The model under review builds one solid part; all positions refer to its coordinate system, in mm. Face numbers are marked on the shaded views. A direction names the side the tool comes from. Give positions to 0.01 mm unless a question says otherwise; leave off trailing zeros. Write each loop counter-clockwise with the first axis right and the second up, starting at its lowest first coordinate (ties: lowest second). Pieces come first, ordered by that corner, then holes. Notation, with made-up numbers: M 53,-18.5 L 62,-18.5 A5 ccw 62,-11.5 Z; hole C -4,-33 d4. An arc over 180 degrees is marked long. Write item = value, one per line. Start each with the question number.
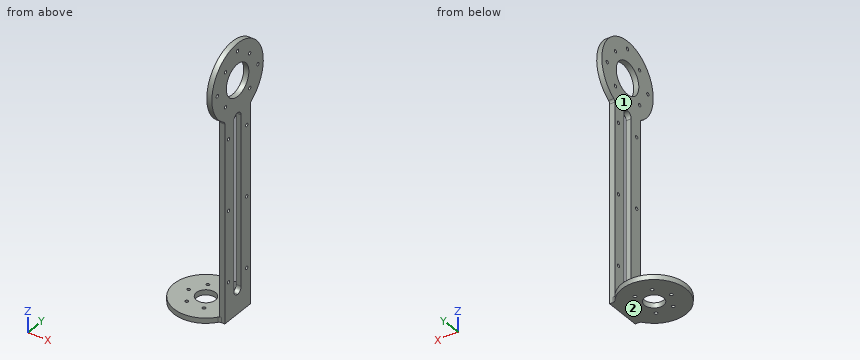
```python
from build123d import *

# Parameters (mm, degrees)
SKETCH_1_R          = 28.5
EXTRUDE_1_DEPTH     = 4
SKETCH_2_R          = 1.25
CUT_EXTRUDE_2_DEPTH = 4
CUT_EXTRUDE_START   = -4
CUT_EXTRUDE_4_DEPTH = 4
SKETCH_5_R          = 7.5
CUT_EXTRUDE_5_DEPTH = 4
SKETCH_6_W          = 4
SKETCH_6_H          = 28.262165522
EXTRUDE_2_DEPTH     = 140
SKETCH_7_R          = 12.5
EXTRUDE_3_DEPTH     = 4
SKETCH_8_R          = 1.25
CUT_EXTRUDE_6_DEPTH = 4
SKETCH_9_R          = 1.25
SKETCH_9_W          = 140
SKETCH_9_H          = 8
CUT_EXTRUDE_7_DEPTH = 4
FILLET_1_R          = 4
FILLET_2_R          = 4
FILLET_3_R          = 2.5


with BuildPart() as part:
    # 草图1 → 凸台-拉伸1 (new body)
    with BuildSketch(Plane.XY):
        Circle(SKETCH_1_R)
    extrude(amount=EXTRUDE_1_DEPTH)

    # 草图2 → 切除-拉伸2 (cut)
    with BuildSketch(Plane.XY.offset(4)):
        with Locations((-13.5, 0)):
            Circle(SKETCH_2_R)
        with Locations((-6.75, 11.691342951)):
            Circle(SKETCH_2_R)
        with Locations((6.75, 11.691342951)):
            Circle(SKETCH_2_R)
        with Locations((6.75, -11.691342951)):
            Circle(SKETCH_2_R)
        with Locations((-6.75, -11.691342951)):
            Circle(SKETCH_2_R)
    extrude(amount=-CUT_EXTRUDE_2_DEPTH, mode=Mode.SUBTRACT)

    # 草图4 → 切除-拉伸4 (cut)
    with BuildSketch(Plane.XY.offset(4).offset(CUT_EXTRUDE_START)):
        with BuildLine():
            ThreePointArc((20.75, -14.131082761), (-25.104780421, 0), (20.75, 14.131082761))
            Line((20.75, 14.131082761), (24.75, 14.131082761))
            ThreePointArc((24.75, 14.131082761), (-28.5, 0), (24.75, -14.131082761))
            Line((24.75, -14.131082761), (20.75, -14.131082761))
        make_face()
        with BuildLine():
            Line((24.75, 14.131082761), (24.75, 0))
            Line((24.75, 0), (28.5, 0))
            ThreePointArc((28.5, 0), (27.546551508, 7.310095759), (24.75, 14.131082761))
        make_face()
        with BuildLine():
            Line((28.5, 0), (24.75, 0))
            Line((24.75, 0), (24.75, -14.131082761))
            ThreePointArc((24.75, -14.131082761), (27.546551508, -7.310095759), (28.5, 0))
        make_face()
    extrude(amount=CUT_EXTRUDE_4_DEPTH, mode=Mode.SUBTRACT)

    # 草图5 → 切除-拉伸5 (cut)
    with BuildSketch(Plane.XY.offset(4)):
        Circle(SKETCH_5_R)
    extrude(amount=-CUT_EXTRUDE_5_DEPTH, mode=Mode.SUBTRACT)

    # 草图6 → 凸台-拉伸2 (add)
    with BuildSketch(Plane.XY.offset(4)):
        with Locations((22.75, 0)):
            Rectangle(SKETCH_6_W, SKETCH_6_H)
    extrude(amount=EXTRUDE_2_DEPTH)

    # 草图7 → 凸台-拉伸3 (add)
    with BuildSketch(Plane(origin=(24.75, 0, 0), x_dir=(0, 0, -1), z_dir=(1, 0, 0))):
        with BuildLine():
            Line((-144, 14.131082761), (-155.25, 14.131082761))
            ThreePointArc((-155.25, 14.131082761), (-208.5, 0), (-155.25, -14.131082761))
            Line((-155.25, -14.131082761), (-144, -14.131082761))
            Line((-144, -14.131082761), (-144, 14.131082761))
        make_face()
        with Locations((-180, 0)):
            Circle(SKETCH_7_R, mode=Mode.SUBTRACT)
    extrude(amount=-EXTRUDE_3_DEPTH)

    # 草图8 → 切除-拉伸6 (cut)
    with BuildSketch(Plane(origin=(24.75, 0, 0), x_dir=(0, 0, -1), z_dir=(1, 0, 0))):
        with Locations((-166.564971157, 13.435028843)):
            Circle(SKETCH_8_R)
        with Locations((-166.564971157, -13.435028843)):
            Circle(SKETCH_8_R)
        with Locations((-193.435028843, -13.435028843)):
            Circle(SKETCH_8_R)
        with Locations((-193.435028843, 13.435028843)):
            Circle(SKETCH_8_R)
    extrude(amount=-CUT_EXTRUDE_6_DEPTH, mode=Mode.SUBTRACT)

    # 草图9 → 切除-拉伸7 (cut)
    with BuildSketch(Plane(origin=(24.75, 0, 0), x_dir=(0, 0, -1), z_dir=(1, 0, 0))):
        with Locations((-140, 10.131082761)):
            Circle(SKETCH_9_R)
        with Locations((-180, 22.5)):
            Circle(SKETCH_9_R)
        with Locations((-202.5, 0)):
            Circle(SKETCH_9_R)
        with Locations((-180, -22.5)):
            Circle(SKETCH_9_R)
        with Locations((-85, 10.131082761)):
            Circle(SKETCH_9_R)
        with Locations((-30, 10.131082761)):
            Circle(SKETCH_9_R)
        with Locations(Location((-30, -10.131082761, 0), (0, 0, 180))):
            Circle(SKETCH_9_R)
        with Locations(Location((-85, -10.131082761, 0), (0, 0, 180))):
            Circle(SKETCH_9_R)
        with Locations(Location((-140, -10.131082761, 0), (0, 0, 180))):
            Circle(SKETCH_9_R)
        with Locations((-85, 0)):
            Rectangle(SKETCH_9_W, SKETCH_9_H)
    extrude(amount=-CUT_EXTRUDE_7_DEPTH, mode=Mode.SUBTRACT)

    # 圆角1
    fillet_1_edges = [part.edges().sort_by_distance(p)[0] for p in [
        (22.75, -4, 155),
        (22.75, 4, 155),
    ]]
    fillet(fillet_1_edges, radius=FILLET_1_R - 0.0001)  # a hair under: the kernel refuses the full size

    # 圆角2
    fillet_2_edges = [part.edges().sort_by_distance(p)[0] for p in [
        (22.75, 4, 15),
        (22.75, -4, 15),
    ]]
    fillet(fillet_2_edges, radius=FILLET_2_R - 0.0001)  # a hair under: the kernel refuses the full size

    # 圆角3
    fillet_3_edges = [part.edges().sort_by_distance(p)[0] for p in [
        (22.75, -14.131082761, 155.25),
        (22.75, 14.131082761, 155.25),
        (20.75, -14.131082761, 2),
        (20.75, 14.131082761, 2),
    ]]
    fillet(fillet_3_edges, radius=FILLET_3_R)


solid = part.part
```
Item 1: Clearance check with flat-ended pins moving along their axes: P1, Ø23.5, axis at x = -8.5, y = 4.5, coming from the +Z side; P2, Ø2, axis at x = 14.5, y = 1, coming from the -Z side; P3, Ø2, axis at x = 22, z = 98, coming from the -Y side; P4, Ø2, axis at y = -18, z = 163.5, coming from the -X side. State where each tip first meets the part, or that it passes through.
Item 2: We need section A-A, the plane z = 105. Write out the cut boundary in (x, y).
Item 3: For the marked faces 1 and 2, list the 3-axis set-ups (+Z, -Z, +X, -X, +Y, -Y) from which the entire face can be reached by the end or side of a thin tool; tool diameter is ignored.
Item 4: To check wall thickness, follow probe 1 along Y at (x, z) = (23.9, 85); probe 2 along X at (y, z) = (15, 179); probe 3 along Z at (x, y) = (-11, 1). State the ranges of each line that lie inside material, in increasing order. Write a range as [from, to].
Item 5: We need section C-C, the plane z = 162. Write out the cut boundary in (x, y), and give its area (3 significant figures).
Item 6: We need section B-B, the plane z = 190. Write out the cut boundary in (x, y).
Worked out:
q1.P1 = 4
q1.P2 = 0
q1.P3 = -14.13
q1.P4 = 20.75
q2.outline = M 20.75,-14.13 L 24.75,-14.13 L 24.75,-4 L 20.75,-4 Z; M 20.75,4 L 24.75,4 L 24.75,14.13 L 20.75,14.13 Z
q3.face_1 = +Z, -X, +Y, -Y
q3.face_2 = -Z, +X, -X, +Y, -Y
q4.probe_1 = [-14.13, -11.38], [-8.88, -4], [4, 8.88], [11.38, 14.13]
q4.probe_2 = [20.75, 24.75]
q4.probe_3 = [0, 4]
q5.outline = M 20.75,-22.1 L 24.75,-22.1 L 24.75,22.1 L 20.75,22.1 Z
q5.area = 177 mm²
q6.outline = M 20.75,-26.69 L 24.75,-26.69 L 24.75,-7.5 L 20.75,-7.5 Z; M 20.75,7.5 L 24.75,7.5 L 24.75,26.69 L 20.75,26.69 Z
